```python
from build123d import *

# Parameters (mm, degrees)
SKETCH_1_R          = 46
EXTRUDE_1_DEPTH     = 3
SKETCH_2_R          = 8
CUT_EXTRUDE_1_DEPTH = 3
SKETCH_3_R          = 2
CUT_EXTRUDE_2_DEPTH = 3


with BuildPart() as part:
    # 스케치1 → 보스-돌출1 (new body)
    with BuildSketch(Plane.XY):
        Circle(SKETCH_1_R)
    extrude(amount=EXTRUDE_1_DEPTH)

    # 스케치2 → 컷-돌출1 (cut)
    with BuildSketch(Plane.XY.offset(3)):
        Circle(SKETCH_2_R)
    extrude(amount=-CUT_EXTRUDE_1_DEPTH, mode=Mode.SUBTRACT)

    # 스케치3 → 컷-돌출2 (cut)
    with BuildSketch(Plane.XY.offset(3)):
        with Locations((-23, 8)):
            Circle(SKETCH_3_R)
        with Locations(Location((-23, -8, 0), (0, 0, 180))):
            Circle(SKETCH_3_R)
        with Locations((23, -8)):
            Circle(SKETCH_3_R)
        with Locations(Location((23, 8, 0), (0, 0, 180))):
            Circle(SKETCH_3_R)
    extrude(amount=-CUT_EXTRUDE_2_DEPTH, mode=Mode.SUBTRACT)


solid = part.part
```
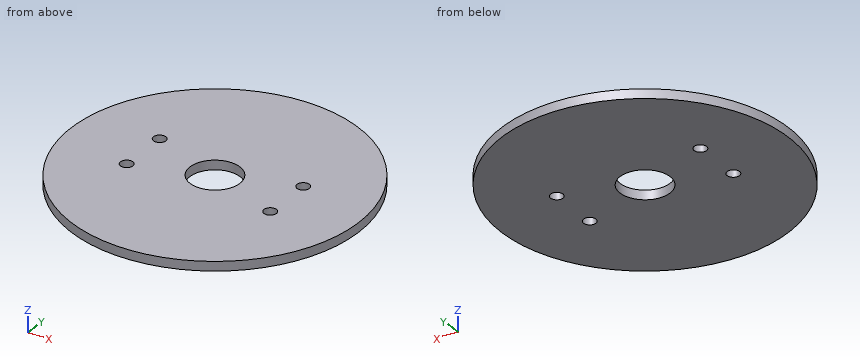
Design review of the part built by this model. Coordinates are the model's own, in mm. Round coordinates to 2 decimals unless told otherwise and drop trailing zeros. Write each loop counter-clockwise with the first axis right and the second up, starting at its lowest first coordinate (ties: lowest second). Pieces come first, ordered by that corner, then holes. Notation, with made-up numbers: (23, -30.75) -> (40, -30.75) arc R31 cw to (40, -5.75) -> close; hole circle Ø3 at (54, -28.75). An arc over 180 degrees is marked (long way). Answer in a Markdown table with one row per item.
Q1. Take a section at B-B, the plane z = 2.1. State the section outline as (x, y) points, then the cut area to 3 significant figures.
The answers:
| item | result |
|---|---|
| outline | circle Ø92 at (0, 0); hole circle Ø4 at (-23, -8); hole circle Ø4 at (-23, 8); hole circle Ø16 at (0, 0); hole circle Ø4 at (23, -8); hole circle Ø4 at (23, 8) |
| area | 6,400 mm² |
Q2. Take a section at A-A, the plane x = 0. State the section outline as (y, z) points, then the cut area to 3 significant figures.
The answers:
| item | result |
|---|---|
| outline | (-46, 0) -> (-8, 0) -> (-8, 3) -> (-46, 3) -> close; (8, 0) -> (46, 0) -> (46, 3) -> (8, 3) -> close |
| area | 228 mm² |
Q3. Clearance check with flat-ended pins moving along their axes: pin 1 Ø1.5 at (x, z) = (-0.5, 1) entering from -Y; pin 2 Ø1.5 at (y, z) = (-3.5, 2.5) entering from +X. State where each tip first meets the part, or that it passes through.
The answers:
| item | result |
|---|---|
| pin 1 | y = -46 |
| pin 2 | x = 45.92 |
Q4. Take a section at D-D, the plane x = 23. State the section outline as (y, z) points, then the cut area to 3 significant figures.
The answers:
| item | result |
|---|---|
| outline | (-39.84, 0) -> (-10, 0) -> (-10, 3) -> (-39.84, 3) -> close; (-6, 0) -> (6, 0) -> (6, 3) -> (-6, 3) -> close; (10, 0) -> (39.84, 0) -> (39.84, 3) -> (10, 3) -> close |
| area | 215 mm² |
Q5. To check wall thickness, follow L1, parallel to Y at x = 0, z = 1.9; L2, parallel to Y at x = -23, z = 1.55; L3, parallel to X at y = 8.5, z = 1.7. State the ranges of each line that lie inside material, in increasing order. Write a range as [from, to].
The answers:
| item | result |
|---|---|
| L1 | [-46, -8], [8, 46] |
| L2 | [-39.84, -10], [-6, 6], [10, 39.84] |
| L3 | [-45.21, -24.94], [-21.06, 21.06], [24.94, 45.21] |
